Source: CAD feature listing. Evaluate the final solid. Frame: model axes, mm. A direction names the side the tool comes from. Round coordinates to 2 decimals unless told otherwise and drop trailing zeros. Order: outer loops, then holes, each group sorted by start corner. A loop starts at its lowest first (then second) coordinate and runs counter-clockwise, first axis right, second up. Notation, with made-up numbers: (3.25, 24) -> (58.25, 24) arc R13 ccw to (58.25, 37) -> close; hole circle Ø9 at (7, -19.5). An arc over 180 degrees is marked (long way). One line per item, written item: value. Start each with the question number.
1) Section B-B (z = 0). Return the cut outline in (x, y).
2) Mould query, pull axis Z, two halves, no side actions, for faces 4 (the face through (6, 1, -20)), 5 (the face through (3, 15.15, 0)), 6 (the face through (2.958, -47.248, 0.478)). Classes: pulls with the +Z half, pulls with the -Z half, needs draft (parallel to the pull), parting line crosses it, or undercut.
3) Section C-C (x = 2.75). State how many separate pieces and enclosed holes the cut face has, and give its area (3 significant figures).
4) Ray query, L1, parallel to Y at x = 1.3, z = 0; L2, parallel to Y at x = 3, z = -26; L3, parallel to Y at x = 4.5, z = 1. Return the intervals inside material, ascending.
5) Pin query (flat end, axial travel): P1, Ø1.6, axis at x = 5.5, z = -14.5, coming from the +Y side; P2, Ø3, axis at y = 32, z = 0, coming from the +X side; P3, Ø1.6, axis at x = 5.5, y = 6.5, coming from the -Z side; P4, Ø5, axis at y = 4.5, z = 35, coming from the -X side. Return the tip coordinate at first contact, or that it passes through.
6) Section A-A (y = 0). Return the cut outline in (x, z).
7) Reachability of faces 1 (the face through (3.04, -25.63, 29.87)), 2 (the face through (4.5, 5, 16)), 3 (the face through (2.958, 47.248, -0.478)) from +Z, -Z, +X, -X, +Y, -Y: full face, straight path, thin tool, end or side. Return the list, or none.
8) Section D-D (z = -26.5). Return the cut outline in (x, y).
```python
from build123d import *

# Parameters (mm, degrees)
SKETCH1_R                = 47.25
BOSS_EXTRUDE1_DEPTH      = 6
CUT_EXTRUDE1_DEPTH       = 20
M5_CLEARANCE_HOLE1_D     = 5.3
M5_CLEARANCE_HOLE1_DEPTH = 16
M5_CLEARANCE_HOLE1_TIP   = 1.59228064
CUT_EXTRUDE2_DEPTH       = 1.5
FILLET1_R                = 1
CUT_EXTRUDE3_DEPTH       = 10


with BuildPart() as part:
    # Sketch1 → Boss-Extrude1 (new body)
    with BuildSketch(Plane(origin=(0, 0, 0), x_dir=(0, 0, -1), z_dir=(1, 0, 0))):
        Circle(SKETCH1_R)
    extrude(amount=BOSS_EXTRUDE1_DEPTH)

    # Sketch2 → Cut-Extrude1 (cut)
    with BuildSketch(Plane(origin=(6, 0, 0), x_dir=(0, 0, -1), z_dir=(1, 0, 0))):
        with BuildLine():
            Line((-12, -12.85), (12, -12.85))
            ThreePointArc((12, -12.85), (12.707106781, -12.557106781), (13, -11.85))
            Line((13, -11.85), (13, -10.85))
            ThreePointArc((13, -10.85), (12.707106781, -11.557106781), (12, -11.85))
            Line((12, -11.85), (-12, -11.85))
            ThreePointArc((-12, -11.85), (-12.707106781, -11.557106781), (-13, -10.85))
            Line((-13, -10.85), (-13, -11.85))
            ThreePointArc((-13, -11.85), (-12.707106781, -12.557106781), (-12, -12.85))
        make_face()
        with BuildLine():
            ThreePointArc((12, -11.85), (12.707106781, -11.557106781), (13, -10.85))
            Line((13, -10.85), (13, -3.85))
            Line((13, -3.85), (13, 14.15))
            ThreePointArc((13, 14.15), (12.707106781, 14.857106781), (12, 15.15))
            Line((12, 15.15), (-12, 15.15))
            ThreePointArc((-12, 15.15), (-12.707106781, 14.857106781), (-13, 14.15))
            Line((-13, 14.15), (-13, -3.85))
            Line((-13, -3.85), (-13, -10.85))
            ThreePointArc((-13, -10.85), (-12.707106781, -11.557106781), (-12, -11.85))
            Line((-12, -11.85), (12, -11.85))
        make_face()
    extrude(amount=-CUT_EXTRUDE1_DEPTH, mode=Mode.SUBTRACT)

    # M5 Clearance Hole1
    with Locations(Plane.ZY):
        with Locations((-32, 0), (0, 32), (32, 0), (0, -32)):
            Hole(M5_CLEARANCE_HOLE1_D / 2, depth=M5_CLEARANCE_HOLE1_DEPTH)
            with Locations((0, 0, -(M5_CLEARANCE_HOLE1_DEPTH + M5_CLEARANCE_HOLE1_TIP / 2))):  # 118° drill point
                Cone(0, M5_CLEARANCE_HOLE1_D / 2, M5_CLEARANCE_HOLE1_TIP, mode=Mode.SUBTRACT)

    # Sketch16 → Cut-Extrude2 (cut)
    with BuildSketch(Plane(origin=(6, 0, 0), x_dir=(0, 0, -1), z_dir=(1, 0, 0))):
        with BuildLine():
            Line((19, -4.85), (19, 15.15))
            Line((19, 15.15), (12, 15.15))
            ThreePointArc((12, 15.15), (12.707106781, 14.857106781), (13, 14.15))
            Line((13, 14.15), (13, -4.85))
            Line((13, -4.85), (19, -4.85))
        make_face()
        with BuildLine():
            ThreePointArc((13, 14.15), (12.707106781, 14.857106781), (12, 15.15))
            Line((12, 15.15), (0, 15.15))
            Line((0, 15.15), (0, -4.85))
            Line((0, -4.85), (13, -4.85))
            Line((13, -4.85), (13, 14.15))
        make_face()
        with BuildLine():
            Line((0, -4.85), (0, 15.15))
            Line((0, 15.15), (-12, 15.15))
            ThreePointArc((-12, 15.15), (-12.707106781, 14.857106781), (-13, 14.15))
            Line((-13, 14.15), (-13, -4.85))
            Line((-13, -4.85), (0, -4.85))
        make_face()
        with BuildLine():
            ThreePointArc((-13, 14.15), (-12.707106781, 14.857106781), (-12, 15.15))
            Line((-12, 15.15), (-19, 15.15))
            Line((-19, 15.15), (-19, -4.85))
            Line((-19, -4.85), (-13, -4.85))
            Line((-13, -4.85), (-13, 14.15))
        make_face()
    extrude(amount=-CUT_EXTRUDE2_DEPTH, mode=Mode.SUBTRACT)

    # Fillet1
    fillet1_edges = [part.edges().sort_by_distance(p)[0] for p in [
        (5.25, -4.85, -19),
        (5.25, 15.15, 19),
        (5.25, 15.15, -19),
        (5.25, -4.85, 19),
    ]]
    fillet(fillet1_edges, radius=FILLET1_R)

    # Sketch17 → Cut-Extrude3 (cut)
    with BuildSketch(Plane(origin=(6, 0, 0), x_dir=(0, 0, -1), z_dir=(1, 0, 0))):
        with BuildLine():
            Line((-20.187898603, -23.723432509), (-21.955665556, -21.955665556))
            Line((-21.955665556, -21.955665556), (-33.410795411, -33.410795411))
            ThreePointArc((-33.410795411, -33.410795411), (-32.332742692, -34.45513387), (-31.222063558, -35.464704245))
            Line((-31.222063558, -35.464704245), (-20.187898603, -24.43053929))
            ThreePointArc((-20.187898603, -24.43053929), (-20.041451993, -24.076985899), (-20.187898603, -23.723432509))
        make_face()
        with BuildLine():
            Line((-33.410795411, -33.410795411), (-21.955665556, -21.955665556))
            Line((-21.955665556, -21.955665556), (-23.723432509, -20.187898603))
            ThreePointArc((-23.723432509, -20.187898603), (-24.076985899, -20.041451993), (-24.43053929, -20.187898603))
            Line((-24.43053929, -20.187898603), (-35.464704245, -31.222063558))
            ThreePointArc((-35.464704245, -31.222063558), (-34.45513387, -32.332742692), (-33.410795411, -33.410795411))
        make_face()
        with BuildLine():
            Line((33.410795411, -33.410795411), (21.955665556, -21.955665556))
            Line((21.955665556, -21.955665556), (20.187898603, -23.723432509))
            ThreePointArc((20.187898603, -23.723432509), (20.041451993, -24.076985899), (20.187898603, -24.43053929))
            Line((20.187898603, -24.43053929), (31.222063558, -35.464704245))
            ThreePointArc((31.222063558, -35.464704245), (32.332742692, -34.45513387), (33.410795411, -33.410795411))
        make_face()
        with BuildLine():
            Line((23.723432509, -20.187898603), (21.955665556, -21.955665556))
            Line((21.955665556, -21.955665556), (33.410795411, -33.410795411))
            ThreePointArc((33.410795411, -33.410795411), (34.45513387, -32.332742692), (35.464704245, -31.222063558))
            Line((35.464704245, -31.222063558), (24.43053929, -20.187898603))
            ThreePointArc((24.43053929, -20.187898603), (24.076985899, -20.041451993), (23.723432509, -20.187898603))
        make_face()
        with BuildLine():
            Line((20.187898603, 23.723432509), (21.955665556, 21.955665556))
            Line((21.955665556, 21.955665556), (33.410795411, 33.410795411))
            ThreePointArc((33.410795411, 33.410795411), (32.332742692, 34.45513387), (31.222063558, 35.464704245))
            Line((31.222063558, 35.464704245), (20.187898603, 24.43053929))
            ThreePointArc((20.187898603, 24.43053929), (20.041451993, 24.076985899), (20.187898603, 23.723432509))
        make_face()
        with BuildLine():
            Line((33.410795411, 33.410795411), (21.955665556, 21.955665556))
            Line((21.955665556, 21.955665556), (23.723432509, 20.187898603))
            ThreePointArc((23.723432509, 20.187898603), (24.076985899, 20.041451993), (24.43053929, 20.187898603))
            Line((24.43053929, 20.187898603), (35.464704245, 31.222063558))
            ThreePointArc((35.464704245, 31.222063558), (34.45513387, 32.332742692), (33.410795411, 33.410795411))
        make_face()
        with BuildLine():
            Line((-23.723432509, 20.187898603), (-21.955665556, 21.955665556))
            Line((-21.955665556, 21.955665556), (-33.410795411, 33.410795411))
            ThreePointArc((-33.410795411, 33.410795411), (-34.45513387, 32.332742692), (-35.464704245, 31.222063558))
            Line((-35.464704245, 31.222063558), (-24.43053929, 20.187898603))
            ThreePointArc((-24.43053929, 20.187898603), (-24.076985899, 20.041451993), (-23.723432509, 20.187898603))
        make_face()
        with BuildLine():
            Line((-33.410795411, 33.410795411), (-21.955665556, 21.955665556))
            Line((-21.955665556, 21.955665556), (-20.187898603, 23.723432509))
            ThreePointArc((-20.187898603, 23.723432509), (-20.041451993, 24.076985899), (-20.187898603, 24.43053929))
            Line((-20.187898603, 24.43053929), (-31.222063558, 35.464704245))
            ThreePointArc((-31.222063558, 35.464704245), (-32.332742692, 34.45513387), (-33.410795411, 33.410795411))
        make_face()
    extrude(amount=-CUT_EXTRUDE3_DEPTH, mode=Mode.SUBTRACT)


solid = part.part
```
Findings:
1. outline: (0, -47.25) -> (6, -47.25) -> (6, -34.65) -> (0, -34.65) -> close; (0, -29.35) -> (6, -29.35) -> (6, -12.85) -> (0, -12.85) -> close; (0, 15.15) -> (6, 15.15) -> (6, 29.35) -> (0, 29.35) -> close; (0, 34.65) -> (6, 34.65) -> (6, 47.25) -> (0, 47.25) -> close
2. face 4: needs draft
2. face 5: undercut
2. face 6: parting line crosses it
3. separate pieces: 1
3. enclosed holes: 5
3. area: 5,810 mm2
4. L1: -47.25 to -34.65, -29.35 to -12.85, 15.15 to 29.35, 34.65 to 47.25
4. L2: -39.45 to -30.24, -21.76 to 21.76, 30.24 to 39.45
4. L3: -47.24 to -34.45, -29.55 to -12.85, 15.15 to 29.55, 34.45 to 47.24
5. P1: y = 45.22
5. P2: through
5. P3: z = -46.9
5. P4: x = 0
6. outline: (0, -47.25) -> (6, -47.25) -> (6, -34.65) -> (0, -34.65) -> close; (0, -29.35) -> (6, -29.35) -> (6, -19) -> (4.5, -19) -> (4.5, -13) -> (0, -13) -> close; (0, 13) -> (4.5, 13) -> (4.5, 19) -> (6, 19) -> (6, 29.35) -> (0, 29.35) -> close; (0, 34.65) -> (6, 34.65) -> (6, 47.25) -> (0, 47.25) -> close
7. face 1: +X, -X
7. face 2: +X
7. face 3: +X, -X, +Y
8. outline: (0, -39.12) -> (6, -39.12) -> (6, -30.74) -> (0, -30.74) -> close; (0, -22.26) -> (6, -22.26) -> (6, 22.26) -> (0, 22.26) -> close; (0, 30.74) -> (6, 30.74) -> (6, 39.12) -> (0, 39.12) -> close
